Geometry check sheet. Reference: the model listing, model coordinates, mm. Round coordinates to 2 decimals unless told otherwise and drop trailing zeros. Order: outer loops, then holes, each group sorted by start corner. A loop starts at its lowest first (then second) coordinate and runs counter-clockwise, first axis right, second up.
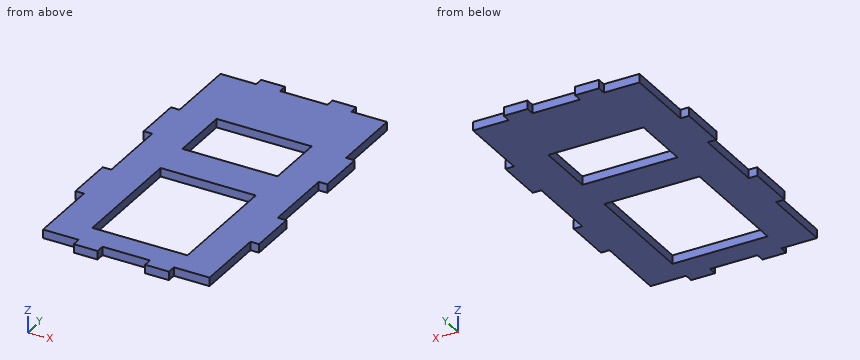
```python
from build123d import *

# Parameters (mm, degrees)
SKETCH1_W           = 98.044
SKETCH1_H           = 174.244
BOSS_EXTRUDE1_DEPTH = 4.572
SKETCH2_W           = 23.622
SKETCH2_H           = 4.572
SKETCH2_W_2         = 25.4
CUT_EXTRUDE1_DEPTH  = 4.572
SKETCH3_W           = 4.572
SKETCH3_H           = 38.1
CUT_EXTRUDE2_DEPTH  = 4.572
SKETCH4_W           = 50.8
SKETCH4_H           = 63.5
SKETCH4_H_2         = 31.75
CUT_EXTRUDE3_DEPTH  = 4.572


with BuildPart() as part:
    # Sketch1 → Boss-Extrude1 (new body)
    with BuildSketch(Plane.XY):
        with Locations((49.022, 87.122)):
            Rectangle(SKETCH1_W, SKETCH1_H)
    extrude(amount=BOSS_EXTRUDE1_DEPTH)

    # Sketch2 → Cut-Extrude1 (cut)
    with BuildSketch(Plane.XY.offset(4.572)):
        with Locations((11.811, 2.286)):
            Rectangle(SKETCH2_W, SKETCH2_H)
        with Locations((49.022, 2.286)):
            Rectangle(SKETCH2_W_2, SKETCH2_H)
        with Locations((86.233, 2.286)):
            Rectangle(SKETCH2_W, SKETCH2_H)
        with Locations((11.811, 171.958)):
            Rectangle(SKETCH2_W, SKETCH2_H)
        with Locations((49.022, 171.958)):
            Rectangle(SKETCH2_W_2, SKETCH2_H)
        with Locations((86.233, 171.958)):
            Rectangle(SKETCH2_W, SKETCH2_H)
    extrude(amount=-CUT_EXTRUDE1_DEPTH, mode=Mode.SUBTRACT)

    # Sketch3 → Cut-Extrude2 (cut)
    with BuildSketch(Plane.XY.offset(4.572)):
        with Locations((2.286, 23.622)):
            Rectangle(SKETCH3_W, SKETCH3_H)
        with Locations((95.758, 23.622)):
            Rectangle(SKETCH3_W, SKETCH3_H)
        with Locations((2.286, 87.122)):
            Rectangle(SKETCH3_W, SKETCH3_H)
        with Locations((2.286, 150.622)):
            Rectangle(SKETCH3_W, SKETCH3_H)
        with Locations((95.758, 150.622)):
            Rectangle(SKETCH3_W, SKETCH3_H)
        with Locations((95.758, 87.122)):
            Rectangle(SKETCH3_W, SKETCH3_H)
    extrude(amount=-CUT_EXTRUDE2_DEPTH, mode=Mode.SUBTRACT)

    # Sketch4 → Cut-Extrude3 (cut)
    with BuildSketch(Plane.XY.offset(4.572)):
        with Locations((49.022, 49.022)):
            Rectangle(SKETCH4_W, SKETCH4_H)
        with Locations((49.022, 116.967)):
            Rectangle(SKETCH4_W, SKETCH4_H_2)
    extrude(amount=-CUT_EXTRUDE3_DEPTH, mode=Mode.SUBTRACT)


solid = part.part
```
(1) Sectioned sample at C-C, the plane z = 2.15. Give the number of separate pieces and of enclosed holes in the cut face, and give its area (3 significant figures).
Returned:
separate pieces: 1
enclosed holes: 2
area: 10,500 mm2
(2) Sectioned sample at A-A, the plane y = 48. Record the cut outline in (x, z).
Returned:
outline: (0, 0) - (23.62, 0) - (23.62, 4.57) - (0, 4.57) - close; (74.42, 0) - (98.04, 0) - (98.04, 4.57) - (74.42, 4.57) - close
(3) Material ranges on line 1 (Y direction, x = 63.5, z = 1); line 2 (Y direction, x = 52.5, z = 2.9); line 3 (X direction, y = 117.5, z = 1.3), recorded low to high.
Returned:
line 1: y = 0 to 17.27, 80.77 to 101.09, 132.84 to 174.24
line 2: y = 4.57 to 17.27, 80.77 to 101.09, 132.84 to 169.67
line 3: x = 0 to 23.62, 74.42 to 98.04
(4) Sectioned sample at B-B, the plane x = 43. Record the cut outline in (y, z).
Returned:
outline: (4.57, 0) - (17.27, 0) - (17.27, 4.57) - (4.57, 4.57) - close; (80.77, 0) - (101.09, 0) - (101.09, 4.57) - (80.77, 4.57) - close; (132.84, 0) - (169.67, 0) - (169.67, 4.57) - (132.84, 4.57) - close
(5) Depth check by flat-ended pin: P1, Ø1.4, axis at y = 1.5, z = 2.5, coming from the -X side; P2, Ø1.4, axis at y = 96.5, z = 3.5, coming from the +X side; P3, Ø2.5, axis at y = 19.5, z = 1.5, coming from the -X side. Enter the tip coordinate at first touch or a pass-through.
Returned:
P1: stops at x = 23.62
P2: stops at x = 93.47
P3: stops at x = 4.57
(6) Sectioned sample at D-D, the plane y = 98. Record the cut outline in (x, z), and give its area (3 significant figures).
Returned:
outline: (4.57, 0) - (93.47, 0) - (93.47, 4.57) - (4.57, 4.57) - close
area: 406 mm2
